Source: CAD feature listing. Evaluate the final solid. Frame: model axes, mm. Round coordinates to 2 decimals unless told otherwise and drop trailing zeros. Order: outer loops, then holes, each group sorted by start corner. A loop starts at its lowest first (then second) coordinate and runs counter-clockwise, first axis right, second up. Notation, with made-up numbers: (37, 80.5) - (54, 80.5) arc R33 ccw to (54, 109.5) - close; hole circle Ø3 at (53, -1.5). An arc over 180 degrees is marked (long way). Return JSON: item names as keys, results as strings. Group by question number.
1) Ray query, line 1 (X direction, y = 3.25, z = 0); line 2 (Y direction, x = 47, z = -2.75); line 3 (X direction, y = -3, z = -0.75). Return the intervals inside material, ascending. Write a range as from..to.
2) Section C-C, the plane x = 224. Return loops of the section in (y, z).
3) Contact query for a flat-ended pin moving along its axis: P1, Ø3, axis at x = 293, z = 3, coming from the -Y side. Output: stop coordinate, or through.
4) Section A-A, the plane z = 0. Return loops of the section in (x, y).
```python
from build123d import *


with BuildPart() as part:
    # Sketch1 → Revolve1 (revolve)
    with BuildSketch(Plane.XY, mode=Mode.PRIVATE) as revolve1_sk:
        with BuildLine():
            Line((0, 2.5), (0, 0))
            Line((0, 0), (490, 0))
            Line((490, 0), (490, 2.5))
            Line((490, 2.5), (489.5, 3))
            Line((489.5, 3), (460.3, 3))
            ThreePointArc((460.3, 3), (460.087867966, 3.087867966), (460, 3.3))
            Line((460, 3.3), (460, 4))
            Line((460, 4), (6, 4))
            Line((6, 4), (6, 3.3))
            ThreePointArc((6, 3.3), (5.912132034, 3.087867966), (5.7, 3))
            Line((5.7, 3), (0.5, 3))
            Line((0.5, 3), (0, 2.5))
        make_face()
    revolve(revolve1_sk.sketch.rotate(Axis((0, 0, 0), (1, 0, 0)), 270), axis=Axis((0, 0, 0), (1, 0, 0)))


solid = part.part
```
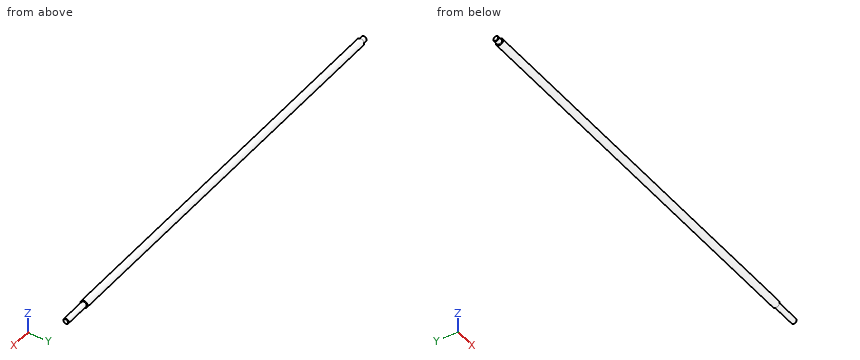
Geometry check:
{
 "1": {"line 1": "6..460", "line 2": "-2.9..2.9", "line 3": "5.92..460.08"},
 "2": {"outline": "circle Ø8 at (0, 0)"},
 "3": {"P1": "y = -3.71"},
 "4": {"outline": "(0, -2.5) - (0.5, -3) - (5.7, -3) arc R0.3 cw to (6, -3.3) - (6, -4) - (460, -4) - (460, -3.3) arc R0.3 cw to (460.3, -3) - (489.5, -3) - (490, -2.5) - (490, 2.5) - (489.5, 3) - (460.3, 3) arc R0.3 cw to (460, 3.3) - (460, 4) - (6, 4) - (6, 3.3) arc R0.3 cw to (5.7, 3) - (0.5, 3) - (0, 2.5) - close"}
}
